from build123d import *

# Parameters (mm, degrees)
BOSS_EXTRUDE1_DEPTH = 60
FILLET1_R           = 20
FILLET2_R           = 30
FILLET3_R           = 10
CUT_EXTRUDE1_REACH  = 143.421
CUT_EXTRUDE2_REACH  = 143.421
SKETCH3_3_R         = 8
SKETCH3_3_R_2       = 6
BOSS_EXTRUDE2_DEPTH = 10
FILLET4_R           = 2


with BuildPart() as part:
    # Sketch1 → Boss-Extrude1 (new, symmetric)
    with BuildSketch(Plane.XY):
        Polygon((0, 0), (100, 0), (100, 20), (20, 20), (20, 100), (0, 100), align=None)
    extrude(amount=BOSS_EXTRUDE1_DEPTH, both=True)

    # Fillet1
    fillet1_edges = [part.edges().sort_by_distance(p)[0] for p in [
        (10, 100, 60),
        (10, 100, -60),
    ]]
    fillet(fillet1_edges, radius=FILLET1_R)

    # Fillet2
    fillet2_edges = [part.edges().sort_by_distance(p)[0] for p in [
        (100, 10, 60),
        (100, 10, -60),
    ]]
    fillet(fillet2_edges, radius=FILLET2_R)

    # Fillet3
    fillet3_edges = [part.edges().sort_by_distance(p)[0] for p in [
        (20, 20, 0),
    ]]
    fillet(fillet3_edges, radius=FILLET3_R)

    # Sketch2 → Cut-Extrude1 (cut, up to next)
    with BuildSketch(Plane(origin=(20, 0, 0), x_dir=(0, 0, -1), z_dir=(1, 0, 0)), mode=Mode.PRIVATE) as cut_extrude1_sk1:
        with BuildLine():
            Line((-40, 86), (40, 86))
            ThreePointArc((40, 86), (46, 80), (40, 74))
            Line((40, 74), (-40, 74))
            ThreePointArc((-40, 74), (-46, 80), (-40, 86))
        make_face()
    cut_extrude1_tool1 = extrude(cut_extrude1_sk1.sketch, amount=-CUT_EXTRUDE1_REACH, mode=Mode.PRIVATE) & part.part
    # Sketch2 → Cut-Extrude1 (cut, up to next)
    with BuildSketch(Plane(origin=(20, 0, 0), x_dir=(0, 0, -1), z_dir=(1, 0, 0)), mode=Mode.PRIVATE) as cut_extrude1_sk2:
        with BuildLine():
            Line((-40, 66), (40, 66))
            ThreePointArc((40, 66), (46, 60), (40, 54))
            Line((40, 54), (-40, 54))
            ThreePointArc((-40, 54), (-46, 60), (-40, 66))
        make_face()
    cut_extrude1_tool2 = extrude(cut_extrude1_sk2.sketch, amount=-CUT_EXTRUDE1_REACH, mode=Mode.PRIVATE) & part.part
    # Sketch2 → Cut-Extrude1 (cut, up to next)
    with BuildSketch(Plane(origin=(20, 0, 0), x_dir=(0, 0, -1), z_dir=(1, 0, 0)), mode=Mode.PRIVATE) as cut_extrude1_sk3:
        with BuildLine():
            Line((-40, 46), (40, 46))
            ThreePointArc((40, 46), (46, 40), (40, 34))
            Line((40, 34), (-40, 34))
            ThreePointArc((-40, 34), (-46, 40), (-40, 46))
        make_face()
    cut_extrude1_tool3 = extrude(cut_extrude1_sk3.sketch, amount=-CUT_EXTRUDE1_REACH, mode=Mode.PRIVATE) & part.part
    add(cut_extrude1_tool1.solids().sort_by_distance((20, 80, 0))[0], mode=Mode.SUBTRACT)
    add(cut_extrude1_tool2.solids().sort_by_distance((20, 60, 0))[0], mode=Mode.SUBTRACT)
    add(cut_extrude1_tool3.solids().sort_by_distance((20, 40, 0))[0], mode=Mode.SUBTRACT)

    # Sketch3 → Cut-Extrude2 (cut, up to next)
    with BuildSketch(Plane(origin=(0, 20, 0), x_dir=(1, 0, 0), z_dir=(0, 1, 0)), mode=Mode.PRIVATE) as cut_extrude2_sk1:
        with BuildLine():
            Line((65, -15), (100, -15))
            Line((100, -15), (100, 15))
            Line((100, 15), (65, 15))
            ThreePointArc((65, 15), (50, 0), (65, -15))
        make_face()
    cut_extrude2_tool1 = extrude(cut_extrude2_sk1.sketch, amount=-CUT_EXTRUDE2_REACH, mode=Mode.PRIVATE) & part.part
    add(cut_extrude2_tool1.solids().sort_by_distance((76.489714, 20, 0))[0], mode=Mode.SUBTRACT)

    # Sketch3_3 → Boss-Extrude2 (add)
    # profile 1 of 2: a face of its own
    with BuildSketch(Plane(origin=(0, 20, 0), x_dir=(1, 0, 0), z_dir=(0, 1, 0))):
        with Locations((70, -30)):
            Circle(SKETCH3_3_R)
        with Locations(Location((70, -30, 0), (0, 0, 180))):
            Circle(SKETCH3_3_R_2, mode=Mode.SUBTRACT)
    # profile 2 of 2: a face of its own
    with BuildSketch(Plane(origin=(0, 20, 0), x_dir=(1, 0, 0), z_dir=(0, 1, 0))):
        with Locations((70, 30)):
            Circle(SKETCH3_3_R)
        with Locations(Location((70, 30, 0), (0, 0, 180))):
            Circle(SKETCH3_3_R_2, mode=Mode.SUBTRACT)
    extrude(amount=BOSS_EXTRUDE2_DEPTH)

    # Fillet4
    fillet4_edges = [part.edges().sort_by_distance(p)[0] for p in [
        (62, 20, 30),
        (62, 20, -30),
    ]]
    fillet(fillet4_edges, radius=FILLET4_R)


solid = part.part
Can you work these out from the model? Positions are in its coordinate system, mm. A direction names the side the tool comes from. Coordinates: 2 decimals unless noted, no trailing zeros. Loops run counter-clockwise (first coordinate to the right, second up) from the corner with the lowest first, then second, coordinate; pieces in that order, holes last. Notation, with made-up numbers: (-36, 80.5) - (6, 80.5) arc R20 ccw to (6, 87.5) - close; hole circle Ø9 at (83, -31). An arc over 180 degrees is marked (long way). Put each result on its own line as item: value. Start each with the question number.
Item 1: If we mould it in two halves opening along Z, with no side actions, what happens to faces 6 (the face through (9.86, 94.297, 53.986)), 7 (the face through (74.76, 24.93, -33.65)), 8 (the face through (20, 72, 1))? For each: +Z half, -Z half, draft (parallel to the pull), parting line (faces both ways), or undercut.
Item 2: Suppose I cut it at A-A (y = 60). Please give me the cut outline in (x, z), and give its area (3 significant figures).
Item 3: Suppose I cut it at B-B (z = -13). Please give me the cut outline in (x, y), and give its area (3 significant figures).
Item 4: Suppose I cut it at D-D (x = 42.5). Please give me the cut outline in (y, z), and give its area (3 significant figures).
Item 5: Which directions (+Z, -Z, +X, -X, +Y, -Y) give clear straight access to the entire face, cutting with the end or side of a thin tool? Please do faces 1 (the face through (83, 10, -15)), 2 (the face through (64.1, 25.9, -35.4)), 3 (the face through (23.01, 22.85, 0.84)), 4 (the face through (0, 51, 1)), 5 (the face through (10, 86, 1)).
Item 6: If I drill on line 1 along Z through (x, y) = (70, 27); line 2 along Y through (x, z) = (8.5, 44.5); line 3 along Y through (x, z) = (37, -52), over which ranges is the centre line in solid material (lowest first)?
Item 7: Suppose I cut it at C-C (x = 10). Please give me the cut outline in (y, z), and give its area (3 significant figures).
Item 8: For pin 1 (3 mm diameter, centred on y = 85, z = 32, fed in from -X); pin 2 (1 mm diameter, centred on y = 66, z = 17.5, fed in from +X); pin 3 (6 mm diameter, centred on x = 80, y = 6.5, fed in from +Z); pin 4 (6 mm diameter, centred on x = 71.5, z = 32.5, fed in from +Y), each with a flat end and sliding along its axis, tell me the tip position at first contact or that it passes through.
Here are the results:
1. face 6: +Z half
1. face 7: undercut
1. face 8: draft
2. outline: (0, -60) - (20, -60) - (20, -46) - (0, -46) - close; (0, 46) - (20, 46) - (20, 60) - (0, 60) - close
2. area: 560 mm²
3. outline: (0, 0) - (57.52, 0) - (57.52, 20) - (30, 20) arc R10 cw to (20, 30) - (20, 34) - (0, 34) - close; (0, 46) - (20, 46) - (20, 54) - (0, 54) - close; (0, 66) - (20, 66) - (20, 74) - (0, 74) - close; (0, 86) - (20, 86) - (20, 100) - (0, 100) - close
3. area: 2,050 mm²
4. outline: (0, -60) - (20, -60) - (20, 60) - (0, 60) - close
4. area: 2,400 mm²
5. face 1: +X, +Y, -Y
5. face 2: +Y
5. face 3: +Z, -Z, +Y
5. face 4: +Z, -Z, -X, +Y, -Y
5. face 5: +X, -X
6. line 1: -38 to -36, -24 to -22, 22 to 24, 36 to 38
6. line 2: 0 to 36.03, 43.97 to 56.03, 63.97 to 76.03, 83.97 to 99.49
6. line 3: 0 to 20
7. outline: (0, -60) - (80, -60) arc R20 ccw to (100, -40) - (100, 40) arc R20 ccw to (80, 60) - (0, 60) - close; hole (34, -40) arc R6 ccw to (46, -40) - (46, 40) arc R6 ccw to (34, 40) - close; hole (54, -40) arc R6 ccw to (66, -40) - (66, 40) arc R6 ccw to (54, 40) - close; hole (74, -40) arc R6 ccw to (86, -40) - (86, 40) arc R6 ccw to (74, 40) - close
7. area: 8,610 mm²
8. pin 1: x = 0
8. pin 2: x = 20
8. pin 3: z = 59.17
8. pin 4: y = 20
